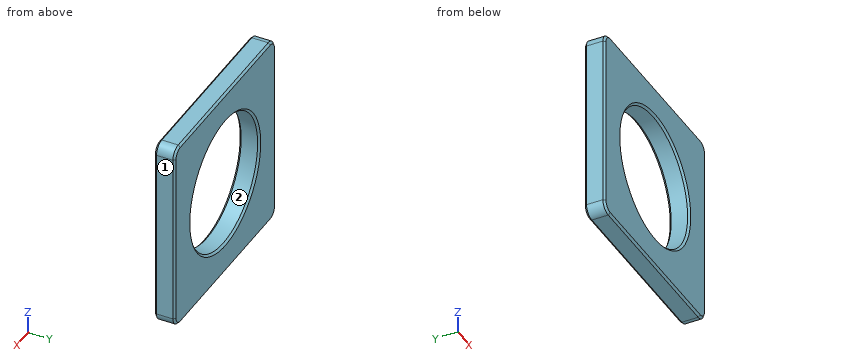
from build123d import *

# Parameters (mm, degrees)
SKETCH1_W           = 95
SKETCH1_H           = 95
SKETCH1_R           = 32.5
BOSS_EXTRUDE1_DEPTH = 10
FILLET1_R           = 5
CHAMFER1_SIZE       = 1


with BuildPart() as part:
    # Sketch1 → Boss-Extrude1 (new body)
    with BuildSketch(Plane(origin=(0, 0, 0), x_dir=(1, 0, 0), z_dir=(0, 1, 0))):
        Rectangle(SKETCH1_W, SKETCH1_H)
        with Locations(Location((0, 0, 0), (0, 0, 270))):
            Circle(SKETCH1_R, mode=Mode.SUBTRACT)
    extrude(amount=BOSS_EXTRUDE1_DEPTH)

    # Fillet1
    fillet1_edges = [part.edges().sort_by_distance(p)[0] for p in [
        (47.5, 5, 47.5),
        (-47.5, 5, 47.5),
        (-47.5, 5, -47.5),
        (47.5, 5, -47.5),
    ]]
    fillet(fillet1_edges, radius=FILLET1_R)

    # Chamfer1
    chamfer1_edges = [part.edges().sort_by_distance(p)[0] for p in [
        (0, 0, -32.5),
        (0, 10, -32.5),
        (-47.5, 0, 0),
        (-47.5, 10, 0),
        (47.5, 0, 0),
        (0, 0, 47.5),
        (0, 0, -47.5),
        (-46.035533906, 0, 46.035533906),
        (46.035533906, 0, 46.035533906),
        (46.035533906, 0, -46.035533906),
        (-46.035533906, 0, -46.035533906),
        (0, 10, -47.5),
        (47.5, 10, 0),
        (0, 10, 47.5),
        (-46.035533906, 10, 46.035533906),
        (46.035533906, 10, 46.035533906),
        (46.035533906, 10, -46.035533906),
        (-46.035533906, 10, -46.035533906),
    ]]
    chamfer(chamfer1_edges, length=CHAMFER1_SIZE)


solid = part.part
Could you check a few things on this model? Use its own coordinates, in mm. Face numbers are marked on the shaded views. Give positions to 0.01 mm unless a question says otherwise; leave off trailing zeros. Order: outer loops, then holes, each group sorted by start corner. A loop starts at its lowest first (then second) coordinate and runs counter-clockwise, first axis right, second up.
Item 1: If we section it at C-C, the plane y = 3.25: Write out the boundary of the cut face in (x, z).
Item 2: If we section it at B-B, the plane z = 0: Write out the boundary of the cut face in (x, y).
Item 3: I need wall thicknesses on line 1 (X direction, y = 7, z = 0); line 2 (X direction, y = 3.25, z = -14); line 3 (Z direction, x = 30, y = 9.25). Which ranges of each line are inside material? Lowest first, please.
Item 4: If we section it at A-A, the plane x = 0: Write out the boundary of the cut face in (y, z), plus the area to 3 significant figures.
Item 5: If we mould it in two halves opening along Z, with no side actions, what happens to the marked faces 1 and 2? For each: pulls with the +Z half, pulls with the -Z half, needs draft (parallel to the pull), parting line crosses it, or undercut.
Item 6: I'm going to push a flat-ended pin straight in: pin 1 (10 mm diameter, centred on x = -16.5, z = 19, fed in from +Y). Where does the tip first touch, or does it pass through?
Values:
1. outline: (-47.5, -42.5) arc R5 ccw to (-42.5, -47.5) - (42.5, -47.5) arc R5 ccw to (47.5, -42.5) - (47.5, 42.5) arc R5 ccw to (42.5, 47.5) - (-42.5, 47.5) arc R5 ccw to (-47.5, 42.5) - close; hole circle Ø65 at (0, 0)
2. outline: (-47.5, 1) - (-46.5, 0) - (-33.5, 0) - (-32.5, 1) - (-32.5, 9) - (-33.5, 10) - (-46.5, 10) - (-47.5, 9) - close; (32.5, 1) - (33.5, 0) - (46.5, 0) - (47.5, 1) - (47.5, 9) - (46.5, 10) - (33.5, 10) - (32.5, 9) - close
3. line 1: x = -47.5 to -32.5, 32.5 to 47.5
3. line 2: x = -47.5 to -29.33, 29.33 to 47.5
3. line 3: z = -47.25 to -13.14, 13.14 to 47.25
4. outline: (0, -46.5) - (1, -47.5) - (9, -47.5) - (10, -46.5) - (10, -33.5) - (9, -32.5) - (1, -32.5) - (0, -33.5) - close; (0, 33.5) - (1, 32.5) - (9, 32.5) - (10, 33.5) - (10, 46.5) - (9, 47.5) - (1, 47.5) - (0, 46.5) - close
4. area: 296 mm2
5. face 1: needs draft
5. face 2: undercut
6. pin 1: passes through
